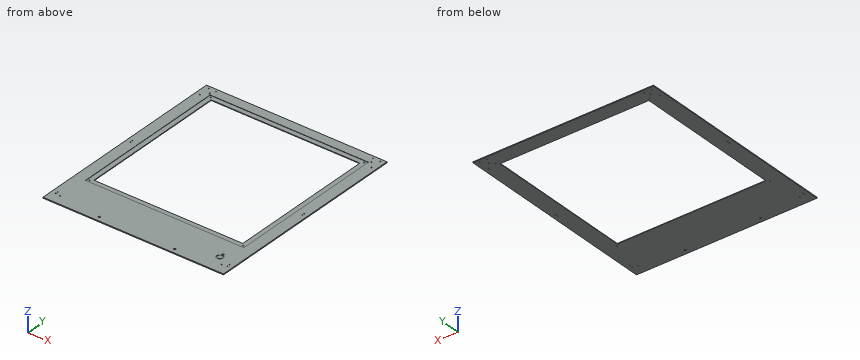
```python
from build123d import *

# Parameters (mm, degrees)
SKETCH005_W     = 570
SKETCH005_H     = 780
PAD001_DEPTH    = 3
SKETCH006_W     = 500
SKETCH006_H     = 500
POCKET004_DEPTH = 1
SKETCH007_R     = 10
SKETCH007_R_2   = 7
POCKET005_DEPTH = 1
SKETCH008_R     = 1.6
POCKET006_DEPTH = 3.001
SKETCH009_W     = 470
SKETCH009_H     = 470
POCKET007_DEPTH = 5
SKETCH030_R     = 1.5
POCKET017_DEPTH = 1935.159379
SKETCH031_R     = 1.5
POCKET018_DEPTH = 5
SKETCH032_R     = 1.5
POCKET019_DEPTH = 2.001
SKETCH033_W     = 606.362244
SKETCH033_H     = 146.592987
POCKET020_DEPTH = 5
SKETCH034_R     = 3
POCKET021_DEPTH = 5


with BuildPart() as part:
    # Sketch005 → Pad001 (new body)
    with BuildSketch(Plane.XY):
        with Locations((0, -110)):
            Rectangle(SKETCH005_W, SKETCH005_H)
    extrude(amount=PAD001_DEPTH)

    # Sketch006 (on Face6 of Pad001) → Pocket004 (cut)
    with BuildSketch(Plane.XY.offset(3)):
        Rectangle(SKETCH006_W, SKETCH006_H)
    extrude(amount=-POCKET004_DEPTH, mode=Mode.SUBTRACT)

    # Sketch007 (on Face5 of Pocket004) → Pocket005 (cut)
    with BuildSketch(Plane.XY.offset(3)):
        with Locations((230, -320)):
            Circle(SKETCH007_R)
        with Locations((230, -320)):
            Circle(SKETCH007_R_2, mode=Mode.SUBTRACT)
        Polygon((230, -301), (226.535898, -307), (233.464102, -307), align=None)
    extrude(amount=-POCKET005_DEPTH, mode=Mode.SUBTRACT)

    # Sketch008 (on Face5 of Pocket005) → Pocket006 (cut, through all)
    with BuildSketch(Plane.XY.offset(3)):
        with Locations((-255, 255)):
            Circle(SKETCH008_R)
        with Locations((255, 255)):
            Circle(SKETCH008_R)
        with Locations((255, -345)):
            Circle(SKETCH008_R)
        with Locations((-255, -345)):
            Circle(SKETCH008_R)
    extrude(amount=-POCKET006_DEPTH, mode=Mode.SUBTRACT)

    # Sketch009 (on Face20 of Pocket006) → Pocket007 (cut)
    with BuildSketch(Plane.XY.offset(2)):
        Rectangle(SKETCH009_W, SKETCH009_H)
    extrude(amount=-POCKET007_DEPTH, mode=Mode.SUBTRACT)

    # Sketch030 (on Face5 of Pocket007) → Pocket017 (cut, through all)
    with BuildSketch(Plane.XY.offset(3)):
        with Locations((-271, 271)):
            Circle(SKETCH030_R)
        with Locations((-247.791107, 271)):
            Circle(SKETCH030_R)
        with Locations((-271, 235.791107)):
            Circle(SKETCH030_R)
        with Locations((-271, -334.320353)):
            Circle(SKETCH030_R)
        with Locations((-271, -342.206532)):
            Circle(SKETCH030_R)
    pocket017 = extrude(amount=-POCKET017_DEPTH, mode=Mode.SUBTRACT)

    # Mirrored: Pocket017 across Sketch030 V_Axis
    add(pocket017.mirror(Plane(origin=(0, 0, 3), x_dir=(0, 0, 1), z_dir=(1, 0, 0))), mode=Mode.SUBTRACT)

    # Sketch031 (on Face1 of CopyClone) → Pocket018 (cut)
    with BuildSketch(Plane(origin=(0, 300, 5), x_dir=(1, 0, 0), z_dir=(0, 0, 1))):
        with Locations((-271, -334.320353)):
            Circle(SKETCH031_R)
        with Locations((-271, -342.206532)):
            Circle(SKETCH031_R)
    pocket018 = extrude(amount=-POCKET018_DEPTH, mode=Mode.SUBTRACT)

    # Mirrored001: Pocket018 across Sketch031 V_Axis
    add(pocket018.mirror(Plane(origin=(0, 300, 5), x_dir=(0, 0, 1), z_dir=(1, 0, 0))), mode=Mode.SUBTRACT)

    # Sketch032 (on Face37 of Mirrored001) → Pocket019 (cut, through all)
    with BuildSketch(Plane.XY.offset(2)):
        with Locations((-242.5, 242.5)):
            Circle(SKETCH032_R)
        with Locations((242.5, 242.5)):
            Circle(SKETCH032_R)
        with Locations((-242.5, -242.5)):
            Circle(SKETCH032_R)
        with Locations((242.5, -242.5)):
            Circle(SKETCH032_R)
    extrude(amount=-POCKET019_DEPTH, mode=Mode.SUBTRACT)

    # Sketch033 (on Face5 of Pocket019) → Pocket020 (cut)
    with BuildSketch(Plane.XY.offset(3)):
        with Locations((-0.325326, -449.115615)):
            Rectangle(SKETCH033_W, SKETCH033_H)
    extrude(amount=-POCKET020_DEPTH, mode=Mode.SUBTRACT)

    # Sketch034 (on Face5 of Pocket020) → Pocket021 (cut)
    with BuildSketch(Plane.XY.offset(3)):
        with Locations((-119.131943, -360.561218)):
            Circle(SKETCH034_R)
        with Locations((119.131943, -360.561218)):
            Circle(SKETCH034_R)
    extrude(amount=-POCKET021_DEPTH, mode=Mode.SUBTRACT)


solid = part.part
```
Design review of the part built by this model. Coordinates are the model's own, in mm. Coordinates: 2 decimals unless noted, no trailing zeros. Order: outer loops, then holes, each group sorted by start corner. A loop starts at its lowest first (then second) coordinate and runs counter-clockwise, first axis right, second up. Notation, with made-up numbers: M 82,9 L 110,9 A20 cw 110,42 Z; hole C 24.5,61 d2. An arc over 180 degrees is marked long. Answer as a JSON object with one key per item and string values. Group by question number.
1) Add section B-B, the plane x = -51. Write out the cut boundary in (y, z), then the cut area to 3 significant figures.
2) Add section C-C, the plane z = 0.75. Count the separate pieces of the cut face and the enclosed holes in it, then the cut area to 3 significant figures.
3) Add section A-A, the plane y = 20. Write out the cut boundary in (x, z), then the cut area to 3 significant figures.
4) Wall thickness on L1, parallel to X at y = 255, z = 1.05; L2, parallel to X at y = 242.5, z = 0.65; L3, parallel to X at y = 37, z = 2.85: over which ranges is each line inside the solid? List them lowest first.
5) For pin 1 (9.5 mm diameter, centred on x = 119.13, y = -360.56, fed in from +Z); pin 2 (1.8 mm diameter, centred on x = 271, y = 271, fed in from -Z); pin 3 (1 mm diameter, centred on x = 180, y = -246, fed in from +Z), all flat-tipped, find the tip position at first contact; note any pin that passes through.
Computed values:
{
 "1": {"outline": "M -375.82,0 L -235,0 L -235,2 L -250,2 L -250,3 L -375.82,3 Z; M 235,0 L 280,0 L 280,3 L 250,3 L 250,2 L 235,2 Z", "area": "527 mm^2"},
 "2": {"separate pieces": "1", "enclosed holes": "25", "area": "153,000 mm^2"},
 "3": {"outline": "M -285,0 L -235,0 L -235,2 L -250,2 L -250,3 L -285,3 Z; M 235,0 L 285,0 L 285,3 L 250,3 L 250,2 L 235,2 Z", "area": "270 mm^2"},
 "4": {"L1": "x = -285 to -256.6, -253.4 to 253.4, 256.6 to 285", "L2": "x = -285 to -244, -241 to 241, 244 to 285", "L3": "x = -285 to -250, 250 to 285"},
 "5": {"pin 1": "stops at z = 3", "pin 2": "passes through", "pin 3": "stops at z = 2"}
}
